Can you work these out from the model? Positions are in its coordinate system, mm. Give positions to 0.01 mm unless a question says otherwise; leave off trailing zeros. Write each loop counter-clockwise with the first axis right and the second up, starting at its lowest first coordinate (ties: lowest second). Pieces come first, ordered by that corner, then holes. Notation, with made-up numbers: (17.25, 28) -> (68.25, 28) arc R35 ccw to (68.25, 66) -> close; hole circle Ø7 at (16, -26.75). An arc over 180 degrees is marked (long way). One line per item, written item: value.
from build123d import *

# Parameters (mm, degrees)
SKETCH1_R             = 3
BOSS_EXTRUDE1_DEPTH   = 1
BOSS_EXTRUDE1_2_DEPTH = 1
BOSS_EXTRUDE1_3_DEPTH = 1
BOSS_EXTRUDE1_4_DEPTH = 1
SKETCH1_W             = 193
SKETCH1_H             = 158
BOSS_EXTRUDE1_5_DEPTH = 1
DELETEFACE1_START     = -1
DELETEFACE1_OUTLINE_R = 3
DELETEFACE1_DEPTH     = 2
SKETCH3_R             = 2.5
CUT_EXTRUDE2_DEPTH    = 384.236219583


with BuildPart() as part:
    # Sketch1 → Boss-Extrude1 (new, symmetric)
    with BuildSketch(Plane.XY):
        with Locations((-372, 55)):
            Circle(SKETCH1_R)
    extrude(amount=BOSS_EXTRUDE1_DEPTH, both=True)


with BuildPart() as body_2:
    # Sketch1 → Boss-Extrude1 2 (new, symmetric)
    with BuildSketch(Plane.XY):
        with Locations(Location((-372, -55, 0), (0, 0, 180))):
            Circle(SKETCH1_R)
    extrude(amount=BOSS_EXTRUDE1_2_DEPTH, both=True)


with BuildPart() as body_3:
    # Sketch1 → Boss-Extrude1 3 (new, symmetric)
    with BuildSketch(Plane.XY):
        with Locations((372, -55)):
            Circle(SKETCH1_R)
    extrude(amount=BOSS_EXTRUDE1_3_DEPTH, both=True)


with BuildPart() as body_4:
    # Sketch1 → Boss-Extrude1 4 (new, symmetric)
    with BuildSketch(Plane.XY):
        with Locations(Location((372, 55, 0), (0, 0, 180))):
            Circle(SKETCH1_R)
    extrude(amount=BOSS_EXTRUDE1_4_DEPTH, both=True)


with BuildPart() as body_5:
    # Sketch1 → Boss-Extrude1 5 (new, symmetric)
    with BuildSketch(Plane.XY):
        Rectangle(SKETCH1_W, SKETCH1_H)
        with Locations((0, 55)):
            Circle(SKETCH1_R, mode=Mode.SUBTRACT)
        with Locations(Location((0, -55, 0), (0, 0, 180))):
            Circle(SKETCH1_R, mode=Mode.SUBTRACT)
    extrude(amount=BOSS_EXTRUDE1_5_DEPTH, both=True)

    # DeleteFace1: read off the stored shape, not the designer's step
    # DeleteFace1 outline → DeleteFace1 (add)
    with BuildSketch(Plane.XY.offset(DELETEFACE1_START)):
        with Locations((0, 55)):
            Circle(DELETEFACE1_OUTLINE_R)
        with Locations((0, -55)):
            Circle(DELETEFACE1_OUTLINE_R)
    extrude(amount=DELETEFACE1_DEPTH)

    # Sketch3 → Cut-Extrude2 (cut, through all)
    with BuildSketch(Plane.XY.offset(1)):
        with Locations(Location((-72, 55, 0), (0, 0, 180))):
            Circle(SKETCH3_R)
        with Locations((72, -55)):
            Circle(SKETCH3_R)
        with Locations((72, 55)):
            Circle(SKETCH3_R)
        with Locations(Location((-72, -55, 0), (0, 0, 180))):
            Circle(SKETCH3_R)
    extrude(amount=-CUT_EXTRUDE2_DEPTH, mode=Mode.SUBTRACT)


solid = body_5.part
1) If we section it at B-B (x = -72): Write out the boundary of the cut face in (y, z), and give its area (3 significant figures).
Answer list:
outline: (-79, -1) -> (-57.5, -1) -> (-57.5, 1) -> (-79, 1) -> close; (-52.5, -1) -> (52.5, -1) -> (52.5, 1) -> (-52.5, 1) -> close; (57.5, -1) -> (79, -1) -> (79, 1) -> (57.5, 1) -> close
area: 296 mm^2
2) We'd pull the mould along Y, two halves only. Please class faces 1 (the face through (70, 53.5, 0)), 2 (the face through (-1, 1, 1)): released by +Y, released by -Y, zero draft, split by the parting line, or undercut.
Answer list:
face 1: undercut
face 2: zero draft
3) I need wall thicknesses on L1, parallel to Y at x = -72, z = 0.4; L2, parallel to X at y = -55.5, z = 0.5; L3, parallel to X at y = 53, z = 0.05. Which ranges of each line are inside material? Lowest first, please.
Answer list:
L1: y = -79 to -57.5, -52.5 to 52.5, 57.5 to 79
L2: x = -96.5 to -74.45, -69.55 to 69.55, 74.45 to 96.5
L3: x = -96.5 to -73.5, -70.5 to 70.5, 73.5 to 96.5
4) Will this pin go through, and if not, where does the flat tip stop? pin 1 (4.5 mm diameter, centred on x = 72, y = 55, fed in from -Z).
Answer list:
pin 1: passes through
5) If we section it at A-A (y = -55): Write out the boundary of the cut face in (x, z).
Answer list:
outline: (-96.5, -1) -> (-74.5, -1) -> (-74.5, 1) -> (-96.5, 1) -> close; (-69.5, -1) -> (69.5, -1) -> (69.5, 1) -> (-69.5, 1) -> close; (74.5, -1) -> (96.5, -1) -> (96.5, 1) -> (74.5, 1) -> close
